from build123d import *

# Parameters (mm, degrees)
SKETCH1_W           = 54
SKETCH1_H           = 106
SKETCH1_W_2         = 49.5
SKETCH1_H_2         = 101.5
BOSS_EXTRUDE1_DEPTH = 5.5
SKETCH2_W           = 54
SKETCH2_H           = 106
SKETCH2_W_2         = 36.2
SKETCH2_H_2         = 48.5
SKETCH2_W_3         = 32
SKETCH2_H_3         = 24
BOSS_EXTRUDE2_DEPTH = 1
BOSS_EXTRUDE3_DEPTH = 2
SKETCH4_R           = 3
BOSS_EXTRUDE4_DEPTH = 2
SKETCH5_R           = 1.1
CUT_EXTRUDE1_DEPTH  = 60.73483071
FILLET1_R           = 3
CHAMFER1_SIZE       = 1
SKETCH6_W           = 49.5
SKETCH6_H           = 1
CUT_EXTRUDE2_DEPTH  = 2


with BuildPart() as part:
    # Sketch1 → Boss-Extrude1 (new body)
    with BuildSketch(Plane(origin=(0, 0, 0), x_dir=(1, 0, 0), z_dir=(0, 1, 0))):
        Rectangle(SKETCH1_W, SKETCH1_H)
        Rectangle(SKETCH1_W_2, SKETCH1_H_2, mode=Mode.SUBTRACT)
    extrude(amount=-BOSS_EXTRUDE1_DEPTH)

    # Sketch2 → Boss-Extrude2 (add)
    with BuildSketch(Plane(origin=(0, 0, 0), x_dir=(1, 0, 0), z_dir=(0, 1, 0))):
        Rectangle(SKETCH2_W, SKETCH2_H)
        with Locations((0, 21.55)):
            Rectangle(SKETCH2_W_2, SKETCH2_H_2, mode=Mode.SUBTRACT)
        with Locations((0, -32)):
            Rectangle(SKETCH2_W_3, SKETCH2_H_3, mode=Mode.SUBTRACT)
    extrude(amount=BOSS_EXTRUDE2_DEPTH)

    # Sketch3 → Boss-Extrude3 (add)
    with BuildSketch(Plane.XZ):
        Polygon((21.5, 11.5715), (17.5, 11.5715), (17.5, 15.0715), (25, 15.0715), (25, -52.4285), (-25, -52.4285), (-25, 15.0715), (-17.5, 15.0715), (-17.5, 11.5715), (-21.5, 11.5715), (-21.5, -48.9285), (21.5, -48.9285), align=None)
    extrude(amount=BOSS_EXTRUDE3_DEPTH)

    # Sketch4 → Boss-Extrude4 (add)
    with BuildSketch(Plane.XZ):
        with Locations((-22, 32.4)):
            Circle(SKETCH4_R)
    boss_extrude4 = extrude(amount=BOSS_EXTRUDE4_DEPTH)

    # Sketch5 → Cut-Extrude1 (cut, symmetric)
    with BuildSketch(Plane.XZ):
        with Locations(Location((-22, 32.4, 0), (0, 0, 270))):
            Circle(SKETCH5_R)
    cut_extrude1 = extrude(amount=CUT_EXTRUDE1_DEPTH, both=True, mode=Mode.SUBTRACT)

    # Mirror1: Boss-Extrude4, Cut-Extrude1 across plane
    add(boss_extrude4.mirror(Plane(origin=(0, 0, 0), x_dir=(0, 0, 1), z_dir=(1, 0, 0))))
    add(cut_extrude1.mirror(Plane(origin=(0, 0, 0), x_dir=(0, 0, 1), z_dir=(1, 0, 0))), mode=Mode.SUBTRACT)

    # Fillet1
    fillet1_edges = [part.edges().sort_by_distance(p)[0] for p in [
        (-27, -2.25, -53),
        (27, -2.25, -53),
        (27, -2.25, 53),
        (-27, -2.25, 53),
    ]]
    fillet(fillet1_edges, radius=FILLET1_R)

    # Chamfer1
    chamfer1_edges = [part.edges().sort_by_distance(p)[0] for p in [
        (-22, 1, 33.5),
        (22, 1, 33.5),
    ]]
    chamfer(chamfer1_edges, length=CHAMFER1_SIZE)

    # Sketch6 → Cut-Extrude2 (cut)
    with BuildSketch(Plane.XZ.offset(5.5)):
        with Locations((0, 51.25)):
            Rectangle(SKETCH6_W, SKETCH6_H)
    extrude(amount=-CUT_EXTRUDE2_DEPTH, mode=Mode.SUBTRACT)


solid = part.part
Can you work these out from the model? Positions are in its coordinate system, mm. A direction names the side the tool comes from. Coordinates: 2 decimals unless noted, no trailing zeros. Write each loop counter-clockwise with the first axis right and the second up, starting at its lowest first coordinate (ties: lowest second). Pieces come first, ordered by that corner, then holes. Notation, with made-up numbers: M -23.5,-23 L 15.5,-23 A9 ccw 15.5,-6 Z; hole C 14,38.25 d10. An arc over 180 degrees is marked long. Use one line per item in the form item = value.
Q1. For P1, Ø12, axis at x = -12, z = -31.5, coming from the +Y side, with a flat end and sliding along its axis, tell me the tip position at first contact or that it passes through.
Model answer:
P1 = through
Q2. If we section it at B-B (z = -17.5): Write out the boundary of the cut face in (x, y).
Model answer:
outline = M -27,-5.5 L -24.75,-5.5 L -24.75,-2 L -21.5,-2 L -21.5,0 L -18.1,0 L -18.1,1 L -27,1 Z; M 18.1,0 L 21.5,0 L 21.5,-2 L 24.75,-2 L 24.75,-5.5 L 27,-5.5 L 27,1 L 18.1,1 Z
Q3. If we section it at A-A (x = 2): Write out the boundary of the cut face in (y, z), then the cut area to 3 significant figures.
Model answer:
outline = M -5.5,-53 L 1,-53 L 1,-45.8 L 0,-45.8 L 0,-48.93 L -2,-48.93 L -2,-50.75 L -5.5,-50.75 Z; M -5.5,51.75 L -3.5,51.75 L -3.5,50.75 L 0,50.75 L 0,44 L 1,44 L 1,53 L -5.5,53 Z; M 0,2.7 L 1,2.7 L 1,20 L 0,20 Z
area = 59.9 mm^2
Q4. If we section it at C-C (z = 32.4): Write out the boundary of the cut face in (x, y), then the cut area to 4 significant figures.
Model answer:
outline = M -27,-5.5 L -24.75,-5.5 L -24.75,-2 L -23.1,-2 L -23.1,0 L -24.1,1 L -27,1 Z; M -20.9,-2 L -19,-2 L -19,0 L -16,0 L -16,1 L -19.9,1 L -20.9,0 Z; M 16,0 L 19,0 L 19,-2 L 20.9,-2 L 20.9,0 L 19.9,1 L 16,1 Z; M 23.1,-2 L 24.75,-2 L 24.75,-5.5 L 27,-5.5 L 27,1 L 24.1,1 L 23.1,0 Z
area = 54.55 mm^2
Q5. For faces 1 (the flat face through (24.75, -3, 0)), 2 (the cylindrical face through (23.074, -1.014, 32.638)), which set-ups out of +Z, -Z, +X, -X, +Y, -Y let a thin tool reach every point of the face, with its end or its side?
Model answer:
face_1 = -Y
face_2 = +Y, -Y
Q6. I need wall thicknesses on line 1 along X through (y, z) = (-0.6, 32.4); line 2 along Z through (x, y) = (23, -4.5); line 3 along X through (y, z) = (-4.75, -36). Which ranges of each line are inside material? Lowest first, please. Write a range as from..to.
Model answer:
line_1 = -27..-23.1, -20.9..-19, 19..20.9, 23.1..27
line_2 = -53..-50.75, 51.75..53
line_3 = -27..-24.75, 24.75..27
